The listing builds one solid part. Answer for the finished solid, in the listing's coordinates (mm). A direction names the side the tool comes from. Give positions to 0.01 mm unless a question says otherwise; leave off trailing zeros. Loops run counter-clockwise (first coordinate to the right, second up) from the corner with the lowest first, then second, coordinate; pieces in that order, holes last.
Item 1: Section A-A, the plane x = 5.08 is taken. Give the vertices of the cut face in (y, z) (3 decimals), and give its area (3 significant figures).
Item 2: A tool of negligible diameter and unlimited length cuts with its end or side. For faces 1 (the face through (53, -3, 34.29)), 2 (the face through (30, -3, 0)), from which of +Z, -Z, +X, -X, +Y, -Y can it reach the whole face along a straight path? Write none if from no direction.
Item 3: This flat-tipped pin is pushed along its axis until it touches: pin 1 Ø3 at (y, z) = (-2, 49.5) entering from -X. Where does it stop, or does it pass through?
Item 4: Consider line 1 along Z through (x, y) = (53, -1.5); line 2 along Y through (x, z) = (5, 68); line 3 along X through (y, z) = (-3.75, 50.5). Determine where each line is inside the solid, lowest interval first.
Item 5: The mould has two halves that part along Y. Classify faces 3 (the face through (30, -6.35, 44)), 4 (the face through (30, 0, 44)), 5 (the face through (0, -3, 43)), 6 (the face through (4.072, -3.948, 42.575)): pulls with the +Y half, pulls with the -Y half, needs draft (parallel to the pull), parting line crosses it, or undercut.
from build123d import *

# Parameters (mm, degrees)
F0_W     = 60.0075
F0_H     = 86.36
F0_W_2   = 3.81
F0_H_2   = 3.81
F1_DEPTH = 6.35
F2_R     = 1.27
F3_DEPTH = 86.361


with BuildPart() as f1:
    # F0 (on Front) → F1 (new body)
    with BuildSketch(Plane.XZ):
        with Locations((30.00375, 43.18)):
            Rectangle(F0_W, F0_H)
        with Locations((52.705, 36.195)):
            Rectangle(F0_W_2, F0_H_2, mode=Mode.SUBTRACT)
        with Locations((52.705, 50.165)):
            Rectangle(F0_W_2, F0_H_2, mode=Mode.SUBTRACT)
    extrude(amount=F1_DEPTH)

    # F2 (on Top) → F3 (cut, through all)
    with BuildSketch(Plane.XY):
        with Locations((5.08, -3.175)):
            Circle(F2_R)
    extrude(amount=F3_DEPTH, mode=Mode.SUBTRACT)


solid = f1.part
Worked answers:
1. outline: (-6.35, 0) - (-4.445, 0) - (-4.445, 86.36) - (-6.35, 86.36) - close; (-1.905, 0) - (0, 0) - (0, 86.36) - (-1.905, 86.36) - close
1. area: 329 mm2
2. face 1: +Y, -Y
2. face 2: -Z, +X, -X, +Y, -Y
3. pin 1: stops at x = 0
4. line 1: z = 0 to 34.29, 38.1 to 48.26, 52.07 to 86.36
4. line 2: y = -6.35 to -4.44, -1.91 to 0
4. line 3: x = 0 to 3.95, 6.21 to 50.8, 54.61 to 60.01
5. face 3: pulls with the -Y half
5. face 4: pulls with the +Y half
5. face 5: needs draft
5. face 6: undercut
